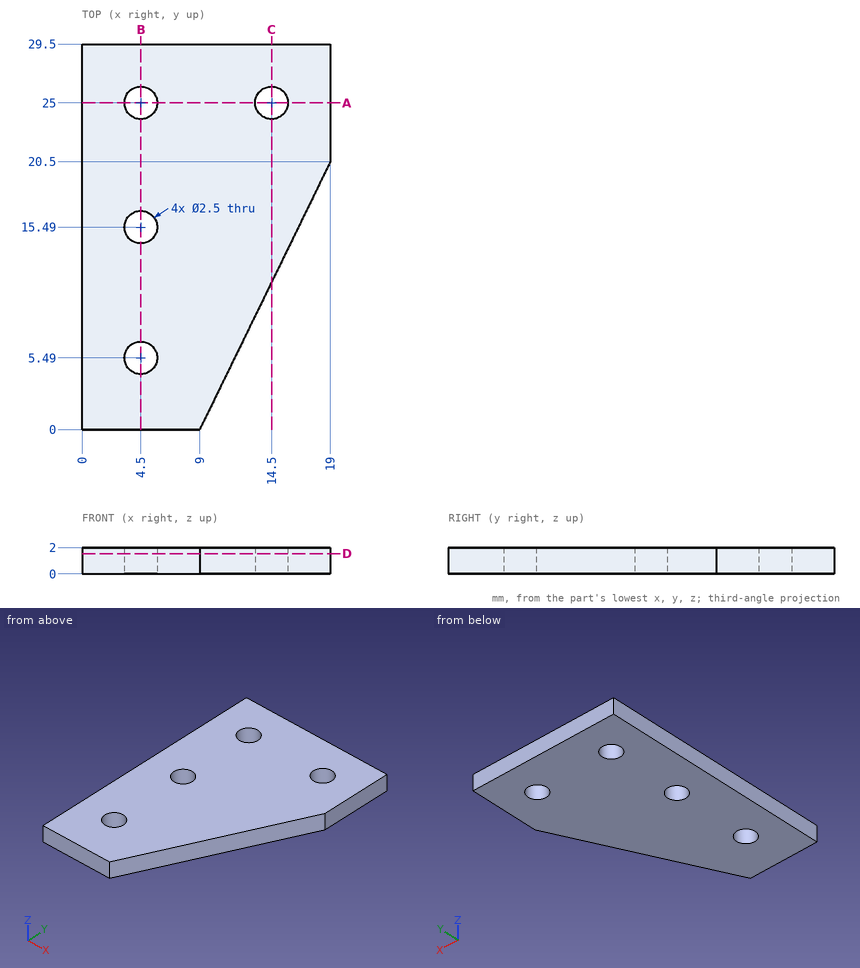
Design review of the part shown in the three views and the two pictorial views. Dimensions are in mm from the part's minimum x, y and z. Round coordinates to 2 decimals unless told otherwise and drop trailing zeros. Loops run counter-clockwise (first coordinate to the right, second up) from the corner with the lowest first, then second, coordinate; pieces in that order, holes last.
Q1. To check wall thickness, follow line 1 along Y through (x, z) = (4.5, 0.6); line 2 along X through (y, z) = (5, 0.8); line 3 along Y through (x, z) = (13.5, 1.6) (3 decimals). State the ranges of each line that lie inside material, in increasing order.
Result sheet:
line 1: y = 0 to 4.24, 6.74 to 14.24, 16.74 to 23.75, 26.25 to 29.5
line 2: x = 0 to 3.35, 5.65 to 11.44
line 3: y = 9.225 to 24.25, 25.75 to 29.5
Q2. Insertion check: pin 1 Ø2 at (x, y) = (4.5, 15.49) entering from +Z; pin 2 Ø1 at (y, z) = (17.5, 0.5) entering from +X. Each pin has a flat end and moves straight along its axis. Give the tip position at first contact, or say it passes through.
Result sheet:
pin 1: passes through
pin 2: stops at x = 17.78
Q3. Add section D-D on z = 1.55. Write out the cut boundary in (x, y), plus the area to 3 significant figures.
Result sheet:
outline: (0, 0) - (9, 0) - (19, 20.5) - (19, 29.5) - (0, 29.5) - close; hole circle Ø2.5 at (4.5, 5.49); hole circle Ø2.5 at (4.5, 15.49); hole circle Ø2.5 at (4.5, 25); hole circle Ø2.5 at (14.5, 25)
area: 438 mm2
Q4. Add section C-C on x = 14.5. Write out the cut boundary in (y, z) (3 decimals), plus the area to 4 significant figures.
Result sheet:
outline: (11.275, 0) - (23.75, 0) - (23.75, 2) - (11.275, 2) - close; (26.25, 0) - (29.5, 0) - (29.5, 2) - (26.25, 2) - close
area: 31.45 mm2
Q5. Add section A-A on y = 25. Write out the cut boundary in (x, z), plus the area to 3 significant figures.
Result sheet:
outline: (0, 0) - (3.25, 0) - (3.25, 2) - (0, 2) - close; (5.75, 0) - (13.25, 0) - (13.25, 2) - (5.75, 2) - close; (15.75, 0) - (19, 0) - (19, 2) - (15.75, 2) - close
area: 28.0 mm2
Q6. Add section B-B on x = 4.5. Write out the cut boundary in (y, z), plus the area to 3 significant figures.
Result sheet:
outline: (0, 0) - (4.24, 0) - (4.24, 2) - (0, 2) - close; (6.74, 0) - (14.24, 0) - (14.24, 2) - (6.74, 2) - close; (16.74, 0) - (23.75, 0) - (23.75, 2) - (16.74, 2) - close; (26.25, 0) - (29.5, 0) - (29.5, 2) - (26.25, 2) - close
area: 44.0 mm2
